Here's how the part is built. I have some questions about the finished solid (model axes, mm). Face numbers are marked on the shaded views. A direction names the side the tool comes from. Coordinates: 2 decimals unless noted, no trailing zeros. Order: outer loops, then holes, each group sorted by start corner. A loop starts at its lowest first (then second) coordinate and runs counter-clockwise, first axis right, second up. Notation, with made-up numbers: (-8, 0.25) - (-2, 0.25) arc R19 cw to (-2, 8.25) - close; hole circle Ø1 at (-39.5, -28.5). An arc over 180 degrees is marked (long way). Answer as CSV lines item,"result". Start each with the question number.
Q1. Suppose I cut it at A-A (y = 0). Please give me the cut outline in (x, z), then the cut area to 3 significant figures.
Q2. I need wall thicknesses on line 1 (Z direction, x = -9.85, y = -11.9); line 2 (X direction, y = -11.4, z = 26.15); line 3 (Z direction, x = 13.5, y = 10.5). Which ranges of each line are inside material? Lowest first, please.
Q3. Suppose I cut it at B-B (x = 10.5). Please give me the cut outline in (y, z).
Q4. Suppose I cut it at C-C (z = 46.5). Please give me the cut outline in (x, y), then the cut area to 3 significant figures.
Q5. For the marked faces 4, 5, 6, 7 and 8, which set-ups out of +Z, -Z, +X, -X, +Y, -Y let a thin tool reach every point of the face, with its end or its side?
Q6. For pin 1 Ø3.5 at (x, z) = (0, 3.15) entering from -Y; pin 2 Ø8.5 at (x, z) = (2.5, 12.5) entering from +Y; pin 3 Ø0.9 at (x, z) = (10, 25.5) entering from -Y; pin 4 Ø2 at (x, y) = (12.5, -13.5) entering from +Z, each with a flat end and sliding along its axis, tell me the tip position at first contact or that it passes through.
Q7. Suppose I cut it at D-D (y = 4). Please give me the cut outline in (x, z), then the cut area to 3 significant figures.
Q8. Thinking about a two-plate mould opening in Z: for the marked faces 1, 2 and 3, which applies, released by +Z, released by -Z, zero draft, split by the parting line, or undercut?
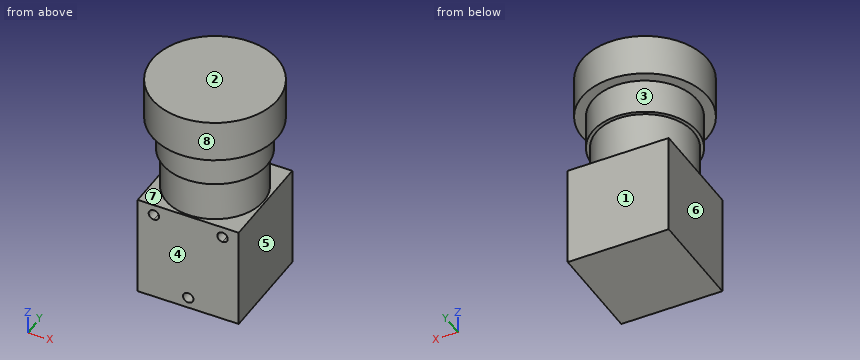
from build123d import *

# Parameters (mm, degrees)
SKETCH_3_W          = 29
SKETCH_3_H          = 29
EXTRUDE_2_DEPTH     = 29.3
SKETCH_4_R          = 14
EXTRUDE_3_DEPTH     = 12
SKETCH_5_R          = 15
EXTRUDE_4_DEPTH     = 10
SKETCH_6_R          = 18
EXTRUDE_5_DEPTH     = 12
CUT_EXTRUDE_1_DEPTH = 5


with BuildPart() as part:
    # 草图3 → 凸台-拉伸2 (new body)
    with BuildSketch(Plane.XY):
        Rectangle(SKETCH_3_W, SKETCH_3_H)
    extrude(amount=EXTRUDE_2_DEPTH)

    # 草图4 → 凸台-拉伸3 (add)
    with BuildSketch(Plane.XY.offset(29.3)):
        Circle(SKETCH_4_R)
    extrude(amount=EXTRUDE_3_DEPTH)

    # 草图5 → 凸台-拉伸4 (add)
    with BuildSketch(Plane.XY.offset(41.3)):
        Circle(SKETCH_5_R)
    extrude(amount=EXTRUDE_4_DEPTH)

    # 草图6 → 凸台-拉伸5 (add)
    with BuildSketch(Plane.XY.offset(51.3)):
        Circle(SKETCH_6_R)
    extrude(amount=EXTRUDE_5_DEPTH)

    # 草图7 → 切除-拉伸1 (cut)
    with BuildSketch(Plane.XZ.offset(14.5)):
        with BuildLine():
            Line((-9.85, 24.65), (-9.85, 26.15))
            Line((-9.85, 26.15), (-8.35, 26.15))
            ThreePointArc((-8.35, 26.15), (-10.910660172, 27.210660172), (-9.85, 24.65))
        make_face()
        with BuildLine():
            Line((-8.35, 26.15), (-9.85, 26.15))
            Line((-9.85, 26.15), (-9.85, 24.65))
            ThreePointArc((-9.85, 24.65), (-8.789339828, 25.089339828), (-8.35, 26.15))
        make_face()
        with BuildLine():
            ThreePointArc((11.35, 26.15), (9.85, 27.65), (8.35, 26.15))
            Line((8.35, 26.15), (9.85, 26.15))
            Line((9.85, 26.15), (9.85, 24.65))
            ThreePointArc((9.85, 24.65), (10.910660172, 25.089339828), (11.35, 26.15))
        make_face()
        with BuildLine():
            Line((9.85, 26.15), (8.35, 26.15))
            ThreePointArc((8.35, 26.15), (8.789339828, 25.089339828), (9.85, 24.65))
            Line((9.85, 24.65), (9.85, 26.15))
        make_face()
        with BuildLine():
            ThreePointArc((1.5, 3.15), (0, 4.65), (-1.5, 3.15))
            Line((-1.5, 3.15), (1.5, 3.15))
        make_face()
        with BuildLine():
            Line((1.5, 3.15), (-1.5, 3.15))
            ThreePointArc((-1.5, 3.15), (0, 1.65), (1.5, 3.15))
        make_face()
    extrude(amount=-CUT_EXTRUDE_1_DEPTH, mode=Mode.SUBTRACT)


solid = part.part
Here are the results:
1,outline,"(-18, 51.3) - (-15, 51.3) - (-15, 41.3) - (-14, 41.3) - (-14, 29.3) - (-14.5, 29.3) - (-14.5, 0) - (14.5, 0) - (14.5, 29.3) - (14, 29.3) - (14, 41.3) - (15, 41.3) - (15, 51.3) - (18, 51.3) - (18, 63.3) - (-18, 63.3) - close"
1,area,"1,920 mm²"
2,line 1,"z = 0 to 24.65, 27.65 to 29.3, 51.3 to 63.3"
2,line 2,"x = -14.5 to -11.35, -8.35 to 8.35, 11.35 to 14.5"
2,line 3,"z = 0 to 29.3, 51.3 to 63.3"
3,outline,"(-14.62, 51.3) - (-10.71, 51.3) - (-10.71, 41.3) - (-9.26, 41.3) - (-9.26, 29.3) - (-14.5, 29.3) - (-14.5, 27.5) - (-9.5, 27.5) - (-9.5, 24.8) - (-14.5, 24.8) - (-14.5, 0) - (14.5, 0) - (14.5, 29.3) - (9.26, 29.3) - (9.26, 41.3) - (10.71, 41.3) - (10.71, 51.3) - (14.62, 51.3) - (14.62, 63.3) - (-14.62, 63.3) - close"
4,outline,"circle Ø30 at (0, 0)"
4,area,"707 mm²"
5,face 4,"-Z, +X, -X, -Y"
5,face 5,"-Z, +X, +Y, -Y"
5,face 6,"-Z, -X, +Y, -Y"
5,face 7,"none"
5,face 8,"+Z"
6,pin 1,"stops at y = -14.5"
6,pin 2,"stops at y = 14.5"
6,pin 3,"stops at y = -9.5"
6,pin 4,"stops at z = 63.3"
7,outline,"(-17.55, 51.3) - (-14.46, 51.3) - (-14.46, 41.3) - (-13.42, 41.3) - (-13.42, 29.3) - (-14.5, 29.3) - (-14.5, 0) - (14.5, 0) - (14.5, 29.3) - (13.42, 29.3) - (13.42, 41.3) - (14.46, 41.3) - (14.46, 51.3) - (17.55, 51.3) - (17.55, 63.3) - (-17.55, 63.3) - close"
7,area,"1,880 mm²"
8,face 1,"zero draft"
8,face 2,"released by +Z"
8,face 3,"undercut"
